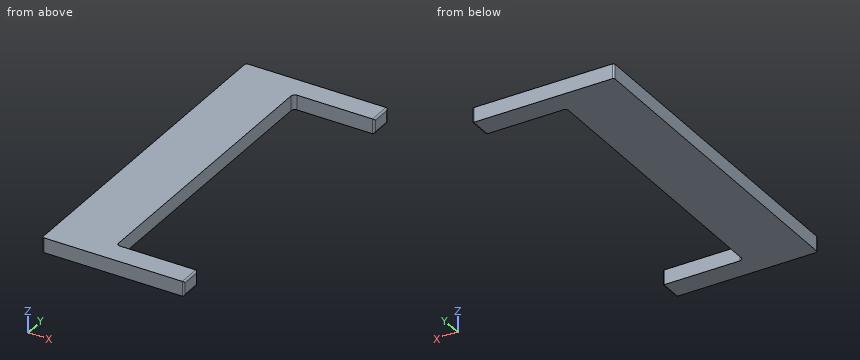
from build123d import *

# Parameters (mm, degrees)
BOSS_EXTRUDE1_DEPTH = 101.6
FILLET1_R           = 25.4
FILLET2_R           = 12.7


with BuildPart() as part:
    # Sketch1 → Boss-Extrude1 (new body)
    with BuildSketch(Plane.XY):
        Polygon((977.9, -152.4), (419.1, -152.4), (419.1, -2159), (977.9, -2159), (977.9, -2311.4), (0, -2311.4), (0, 0), (977.9, 0), align=None)
    extrude(amount=BOSS_EXTRUDE1_DEPTH)

    # Fillet1
    fillet1_edges = [part.edges().sort_by_distance(p)[0] for p in [
        (419.1, -152.4, 50.8),
        (419.1, -2159, 50.8),
    ]]
    fillet(fillet1_edges, radius=FILLET1_R)

    # Fillet2
    fillet2_edges = [part.edges().sort_by_distance(p)[0] for p in [
        (977.9, -2235.2, 101.6),
        (0, 0, 50.8),
        (977.9, 0, 50.8),
        (977.9, -152.4, 50.8),
        (977.9, -2159, 50.8),
        (977.9, -2311.4, 50.8),
        (0, -2311.4, 50.8),
        (977.9, -76.2, 101.6),
        (977.9, -76.2, 0),
        (977.9, -2235.2, 0),
    ]]
    fillet(fillet2_edges, radius=FILLET2_R)


solid = part.part
The listing builds one solid part. Answer for the finished solid, in the listing's coordinates (mm). Round coordinates to 2 decimals unless told otherwise and drop trailing zeros. Write each loop counter-clockwise with the first axis right and the second up, starting at its lowest first coordinate (ties: lowest second). Pieces come first, ordered by that corner, then holes. Notation, with made-up numbers: (-32, 11) - (-4, 11) arc R27 cw to (-4, 37) - close; hole circle Ø3 at (5.5, 4). An arc over 180 degrees is marked (long way). Use one line per item in the form item = value. Start each with the question number.
Item 1: A cutting plane is placed at A-A (x = 797). Write down the section's boundary in (y, z).
Item 2: Find the intervals of material crossed by line 1 (Y direction, x = 821.5, z = 43); line 2 (X direction, y = -1144.5, z = 36.5); line 3 (Y direction, x = 438.5, z = 70.5), in increasing order. Write a range as [from, to].
Item 3: A cutting plane is placed at C-C (y = -2106.5). Write down the section's boundary in (x, z).
Item 4: A cutting plane is placed at B-B (z = 45). Write down the section's boundary in (x, y), plus the area to 3 significant figures.
Item 5: A flat-ended cylindrical pin translates along its axis: pin 1 Ø3 at (y, z) = (-1003.5, 11.5) entering from +X. Find the tip coordinate at first contact, or state that the pin passes through.
The answers:
q1.outline = (-2311.4, 0) - (-2159, 0) - (-2159, 101.6) - (-2311.4, 101.6) - close; (-152.4, 0) - (0, 0) - (0, 101.6) - (-152.4, 101.6) - close
q2.line_1 = [-2311.4, -2159], [-152.4, 0]
q2.line_2 = [0, 419.1]
q2.line_3 = [-2311.4, -2158.28], [-153.12, 0]
q3.outline = (0, 0) - (419.1, 0) - (419.1, 101.6) - (0, 101.6) - close
q4.outline = (0, -2298.7) arc R12.7 ccw to (12.7, -2311.4) - (965.2, -2311.4) arc R12.7 ccw to (977.9, -2298.7) - (977.9, -2171.7) arc R12.7 ccw to (965.2, -2159) - (444.5, -2159) arc R25.4 cw to (419.1, -2133.6) - (419.1, -177.8) arc R25.4 cw to (444.5, -152.4) - (965.2, -152.4) arc R12.7 ccw to (977.9, -139.7) - (977.9, -12.7) arc R12.7 ccw to (965.2, 0) - (12.7, 0) arc R12.7 ccw to (0, -12.7) - close
q4.area = 1,140,000 mm^2
q5.pin_1 = 419.1
